Build history of the part. All positions in model axes, mm. Face numbers are marked on the shaded views. A direction names the side the tool comes from. Give positions to 0.01 mm unless a question says otherwise; leave off trailing zeros. Loops run counter-clockwise (first coordinate to the right, second up) from the corner with the lowest first, then second, coordinate; pieces in that order, holes last.
1) Band-saw the part on C-C on z = 0. State how many separate pieces and enclosed holes the cut face has, then the cut area to 3 significant figures.
2) Wall check: line 1 (X direction, y = 0, z = 2.9); line 2 (Y direction, x = 8.8, z = 0); line 3 (X direction, y = 8.5, z = -1.5). Give the ranges that are in metal, low to high.
3) Two-plate mould, pull along Y, no slides. Class the marked faces 6, 7, 8 and 9: +Y half, -Y half, draft (parallel to the pull), parting line (faces both ways), or undercut.
4) Band-saw the part on D-D on y = 10. List the corners of the cut face in (x, z), then the cut area to 3 significant figures.
5) 3-axis set-ups, long thin cutter, end or side, ignore diameter. For the marked faces 1, 2, 3, 4 and 5: which of +Z, -Z, +X, -X, +Y, -Y reach the whole face in a straight line?
6) Flat gauge pins, fed straight in: P1, Ø2.5, axis at y = 10.5, z = 0, coming from the +X side; P2, Ø1.8, axis at x = 14.5, z = -2.5, coming from the +Y side; P3, Ø5, axis at y = 10, z = 0, coming from the -X side. Where does each tip first touch, or does it go through?
7) Band-saw the part on A-A on x = -14. List the corners of the cut face in (y, z), then the cut area to 3 significant figures.
8) Band-saw the part on B-B on y = 0. List the corners of the cut face in (x, z).
```python
from build123d import *

# Parameters (mm, degrees)
SKETCH1_W                      = 22
SKETCH1_H                      = 29
BOSS_EXTRUDE1_DEPTH            = 5
SKETCH3_W                      = 34
SKETCH3_H                      = 10
BOSS_EXTRUDE2_DEPTH            = 5
F_16_0_16_DIAMETER_HOLE1_D     = 16
F_16_0_16_DIAMETER_HOLE1_DEPTH = 6
F_14_0_14_DIAMETER_HOLE1_D     = 14
M3_CLEARANCE_HOLE1_D           = 3.2
SKETCH12_W                     = 2.5
SKETCH12_H                     = 8.112511343
CUT_EXTRUDE1_DEPTH             = 25.779023387
M3X0_5_TAPPED_HOLE1_D          = 2.5
M3X0_5_TAPPED_HOLE1_DEPTH      = 9.75
CBORE_FOR_M3_SHCS1_D           = 3.2
CBORE_FOR_M3_SHCS1_DEPTH       = 9.75
CBORE_FOR_M3_SHCS1_CBORE_D     = 6.5
CBORE_FOR_M3_SHCS1_CBORE_DEPTH = 3
CHAMFER1_SIZE                  = 0.5


with BuildPart() as part:
    # Sketch1 → Boss-Extrude1 (new, symmetric)
    with BuildSketch(Plane.XY):
        with Locations((0, 0.5)):
            Rectangle(SKETCH1_W, SKETCH1_H)
    extrude(amount=BOSS_EXTRUDE1_DEPTH, both=True)

    # Sketch3 → Boss-Extrude2 (add)
    with BuildSketch(Plane.XZ.offset(14)):
        Rectangle(SKETCH3_W, SKETCH3_H)
    extrude(amount=-BOSS_EXTRUDE2_DEPTH)

    # Ø16.0 (16) Diameter Hole1
    with Locations(Plane(origin=(0, 0, -5), x_dir=(-1, 0, 0), z_dir=(0, 0, -1))):
        with Locations((0, 0)):
            Hole(F_16_0_16_DIAMETER_HOLE1_D / 2, depth=F_16_0_16_DIAMETER_HOLE1_DEPTH)

    # Ø14.0 (14) Diameter Hole1 (through all)
    with Locations(Plane(origin=(0, 0, 1), x_dir=(-1, 0, 0), z_dir=(0, 0, -1))):
        with Locations((0, 0)):
            Hole(F_14_0_14_DIAMETER_HOLE1_D / 2)

    # M3 Clearance Hole1 (through all)
    with Locations(Plane(origin=(0, -9, 0), x_dir=(1, 0, 0), z_dir=(0, 1, 0))):
        with Locations((-14, 0), (14, 0)):
            Hole(M3_CLEARANCE_HOLE1_D / 2)

    # Sketch12 → Cut-Extrude1 (cut, through all)
    with BuildSketch(Plane.XY.offset(5)):
        with Locations((0, 10.943744329)):
            Rectangle(SKETCH12_W, SKETCH12_H)
    extrude(amount=-CUT_EXTRUDE1_DEPTH, mode=Mode.SUBTRACT)

    # M3x0.5 Tapped Hole1
    with Locations(Plane.ZY.offset(11)):
        with Locations((0, 10)):
            Hole(M3X0_5_TAPPED_HOLE1_D / 2, depth=M3X0_5_TAPPED_HOLE1_DEPTH)

    # CBORE for M3 SHCS1
    with Locations(Plane(origin=(11, 0, 0), x_dir=(0, 0, -1), z_dir=(1, 0, 0))):
        with Locations((0, 10)):
            CounterBoreHole(CBORE_FOR_M3_SHCS1_D / 2, CBORE_FOR_M3_SHCS1_CBORE_D / 2, CBORE_FOR_M3_SHCS1_CBORE_DEPTH, depth=CBORE_FOR_M3_SHCS1_DEPTH)

    # Chamfer1
    chamfer1_edges = [part.edges().sort_by_distance(p)[0] for p in [
        (0, -7, 5),
        (0, -8, -5),
        (-11, 10, 1.25),
    ]]
    chamfer(chamfer1_edges, length=CHAMFER1_SIZE)


solid = part.part
```
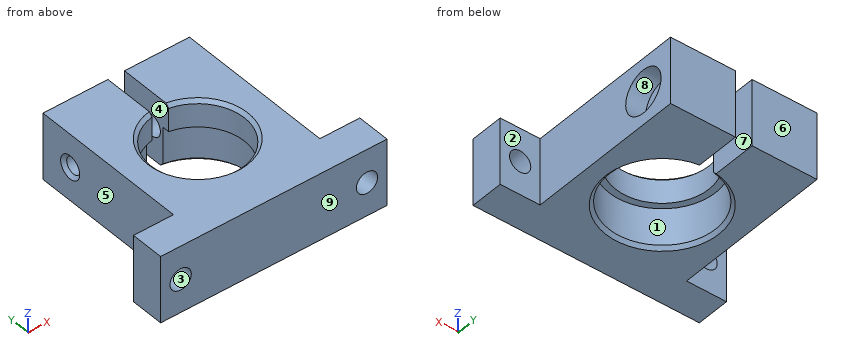
Findings below:
1. separate pieces: 5
1. enclosed holes: 0
1. area: 382 mm2
2. line 1: x = -11 to -7, 7 to 11
2. line 2: y = -14 to 6.75, 13.25 to 15
2. line 3: x = -11 to -1.25, 1.25 to 8
3. face 6: +Y half
3. face 7: draft
3. face 8: undercut
3. face 9: -Y half
4. outline: (-11, -5) - (-1.25, -5) - (-1.25, -1.25) - (-10.5, -1.25) - (-11, -1.75) - close; (-11, 1.75) - (-10.5, 1.25) - (-1.25, 1.25) - (-1.25, 5) - (-11, 5) - close; (1.25, -5) - (11, -5) - (11, -3.25) - (8, -3.25) - (8, -1.6) - (1.25, -1.6) - close; (1.25, 1.6) - (8, 1.6) - (8, 3.25) - (11, 3.25) - (11, 5) - (1.25, 5) - close
4. area: 129 mm2
5. face 1: -Z
5. face 2: +Z, -Z, +X, +Y
5. face 3: +Y, -Y
5. face 4: +Z, -Z, +Y
5. face 5: +Z, -Z, -X, +Y
6. P1: stops at x = 8
6. P2: stops at y = -9
6. P3: stops at x = -11
7. outline: (-14, -5) - (-9, -5) - (-9, -1.6) - (-14, -1.6) - close; (-14, 1.6) - (-9, 1.6) - (-9, 5) - (-14, 5) - close
7. area: 34.0 mm2
8. outline: (-11, -5) - (-8.5, -5) - (-8, -4.5) - (-8, 1) - (-7, 1) - (-7, 4.5) - (-7.5, 5) - (-11, 5) - close; (7, 1) - (8, 1) - (8, -4.5) - (8.5, -5) - (11, -5) - (11, 5) - (7.5, 5) - (7, 4.5) - close
